from build123d import *

# Parameters (mm, degrees)
SKETCH1_W           = 100
SKETCH1_H           = 100
SKETCH1_R           = 11
BOSS_EXTRUDE1_DEPTH = 12
SKETCH9_W           = 100
SKETCH9_H           = 50
BOSS_EXTRUDE3_DEPTH = 12
CUT_EXTRUDE3_REACH  = 114.446
SKETCH4_R           = 10.5
CUT_EXTRUDE4_REACH  = 114.446
CUT_EXTRUDE5_REACH  = 114.446
SKETCH6_R           = 26
CUT_EXTRUDE6_REACH  = 114.446
CUT_EXTRUDE7_REACH  = 114.446
SKETCH11_R          = 52.045454545
CUT_EXTRUDE8_REACH  = 114.446
SKETCH12_R          = 3


with BuildPart() as part:
    # Sketch1 → Boss-Extrude1 (new body)
    with BuildSketch(Plane(origin=(0, 0, 0), x_dir=(1, 0, 0), z_dir=(0, 1, 0))):
        Rectangle(SKETCH1_W, SKETCH1_H)
        with Locations(Location((0, 0, 0), (0, 0, 270))):
            Circle(SKETCH1_R, mode=Mode.SUBTRACT)
    extrude(amount=BOSS_EXTRUDE1_DEPTH)

    # Sketch9 → Boss-Extrude3 (add)
    with BuildSketch(Plane(origin=(0, 12, 0), x_dir=(1, 0, 0), z_dir=(0, 1, 0))):
        with Locations((0, -75)):
            Rectangle(SKETCH9_W, SKETCH9_H)
    extrude(amount=-BOSS_EXTRUDE3_DEPTH)

    # Sketch4 → Cut-Extrude3 (cut, up to next)
    with BuildSketch(Plane(origin=(0, 12, 0), x_dir=(1, 0, 0), z_dir=(0, 1, 0)), mode=Mode.PRIVATE) as cut_extrude3_sk1:
        with Locations(Location((-36, -20, 0), (0, 0, 270))):
            Circle(SKETCH4_R)
    cut_extrude3_tool1 = extrude(cut_extrude3_sk1.sketch, amount=-CUT_EXTRUDE3_REACH, mode=Mode.PRIVATE) & part.part
    # Sketch4 → Cut-Extrude3 (cut, up to next)
    with BuildSketch(Plane(origin=(0, 12, 0), x_dir=(1, 0, 0), z_dir=(0, 1, 0)), mode=Mode.PRIVATE) as cut_extrude3_sk2:
        with Locations(Location((36, -20, 0), (0, 0, 270))):
            Circle(SKETCH4_R)
    cut_extrude3_tool2 = extrude(cut_extrude3_sk2.sketch, amount=-CUT_EXTRUDE3_REACH, mode=Mode.PRIVATE) & part.part
    add(cut_extrude3_tool1.solids().sort_by_distance((-36, 12, 20))[0], mode=Mode.SUBTRACT)
    add(cut_extrude3_tool2.solids().sort_by_distance((36, 12, 20))[0], mode=Mode.SUBTRACT)

    # Sketch5 → Cut-Extrude4 (cut, up to next)
    with BuildSketch(Plane(origin=(0, 12, 0), x_dir=(1, 0, 0), z_dir=(0, 1, 0)), mode=Mode.PRIVATE) as cut_extrude4_sk1:
        Polygon((-50, 0), (-32, 0), (-32, 18), (32, 18), (32, 0), (50, 0), (50, 50), (-50, 50), align=None)
    cut_extrude4_tool1 = extrude(cut_extrude4_sk1.sketch, amount=-CUT_EXTRUDE4_REACH, mode=Mode.PRIVATE) & part.part
    add(cut_extrude4_tool1.solids().sort_by_distance((0, 12, -29.790021))[0], mode=Mode.SUBTRACT)

    # Sketch6 → Cut-Extrude5 (cut, up to next)
    with BuildSketch(Plane(origin=(0, 12, 0), x_dir=(1, 0, 0), z_dir=(0, 1, 0)), mode=Mode.PRIVATE) as cut_extrude5_sk1:
        with Locations(Location((-0.234960822, -55, 0), (0, 0, 270))):
            Circle(SKETCH6_R)
    cut_extrude5_tool1 = extrude(cut_extrude5_sk1.sketch, amount=-CUT_EXTRUDE5_REACH, mode=Mode.PRIVATE) & part.part
    add(cut_extrude5_tool1.solids().sort_by_distance((-0.234961, 12, 55))[0], mode=Mode.SUBTRACT)

    # Sketch10 → Cut-Extrude6 (cut, up to next)
    with BuildSketch(Plane(origin=(0, 12, 0), x_dir=(1, 0, 0), z_dir=(0, 1, 0)), mode=Mode.PRIVATE) as cut_extrude6_sk1:
        with BuildLine():
            Line((-10.234960822, -88.541019662), (-10.234960822, -100))
            Line((-10.234960822, -100), (-50, -100))
            Line((-50, -100), (-50, -40))
            Line((-50, -40), (-35.234177398, -54.765822602))
            ThreePointArc((-35.234177398, -54.765822602), (-28.367208461, -75.822503278), (-10.234960822, -88.541019662))
        make_face()
    cut_extrude6_tool1 = extrude(cut_extrude6_sk1.sketch, amount=-CUT_EXTRUDE6_REACH, mode=Mode.PRIVATE) & part.part
    # Sketch10 → Cut-Extrude6 (cut, up to next)
    with BuildSketch(Plane(origin=(0, 12, 0), x_dir=(1, 0, 0), z_dir=(0, 1, 0)), mode=Mode.PRIVATE) as cut_extrude6_sk2:
        with BuildLine():
            Line((9.765039178, -88.541019662), (9.765039178, -100))
            Line((9.765039178, -100), (50, -100))
            Line((50, -100), (50, -40))
            Line((50, -40), (34.764245164, -55.235754836))
            ThreePointArc((34.764245164, -55.235754836), (27.756864791, -76.010894766), (9.765039178, -88.541019662))
        make_face()
    cut_extrude6_tool2 = extrude(cut_extrude6_sk2.sketch, amount=-CUT_EXTRUDE6_REACH, mode=Mode.PRIVATE) & part.part
    # Sketch10 → Cut-Extrude6 (cut, up to next)
    with BuildSketch(Plane(origin=(0, 12, 0), x_dir=(1, 0, 0), z_dir=(0, 1, 0)), mode=Mode.PRIVATE) as cut_extrude6_sk3:
        with BuildLine():
            Line((-0.734960822, -80.995191863), (-0.734960822, -100))
            Line((-0.734960822, -100), (0.265039178, -100))
            Line((0.265039178, -100), (0.265039178, -80.995191863))
            ThreePointArc((0.265039178, -80.995191863), (-0.234960822, -81), (-0.734960822, -80.995191863))
        make_face()
    cut_extrude6_tool3 = extrude(cut_extrude6_sk3.sketch, amount=-CUT_EXTRUDE6_REACH, mode=Mode.PRIVATE) & part.part
    add(cut_extrude6_tool1.solids().sort_by_distance((-35.978986, 12, 79.410224))[0], mode=Mode.SUBTRACT)
    add(cut_extrude6_tool2.solids().sort_by_distance((35.780347, 12, 79.379296))[0], mode=Mode.SUBTRACT)
    add(cut_extrude6_tool3.solids().sort_by_distance((-0.234961, 12, 90.499199))[0], mode=Mode.SUBTRACT)

    # Sketch11 → Cut-Extrude7 (cut, up to next)
    with BuildSketch(Plane(origin=(0, 12, 0), x_dir=(1, 0, 0), z_dir=(0, 1, 0)), mode=Mode.PRIVATE) as cut_extrude7_sk1:
        with Locations((0, 41.045454545)):
            Circle(SKETCH11_R)
    cut_extrude7_tool1 = extrude(cut_extrude7_sk1.sketch, amount=-CUT_EXTRUDE7_REACH, mode=Mode.PRIVATE) & part.part
    add(cut_extrude7_tool1.solids().sort_by_distance((0, 12, -41.045455))[0], mode=Mode.SUBTRACT)

    # Sketch12 → Cut-Extrude8 (cut, up to next)
    with BuildSketch(Plane(origin=(0, 12, 0), x_dir=(1, 0, 0), z_dir=(0, 1, 0)), mode=Mode.PRIVATE) as cut_extrude8_sk1:
        with Locations(Location((-15.162534268, -20, 0), (0, 0, 270))):
            Circle(SKETCH12_R)
    cut_extrude8_tool1 = extrude(cut_extrude8_sk1.sketch, amount=-CUT_EXTRUDE8_REACH, mode=Mode.PRIVATE) & part.part
    # Sketch12 → Cut-Extrude8 (cut, up to next)
    with BuildSketch(Plane(origin=(0, 12, 0), x_dir=(1, 0, 0), z_dir=(0, 1, 0)), mode=Mode.PRIVATE) as cut_extrude8_sk2:
        with Locations(Location((14.837465732, -20, 0), (0, 0, 270))):
            Circle(SKETCH12_R)
    cut_extrude8_tool2 = extrude(cut_extrude8_sk2.sketch, amount=-CUT_EXTRUDE8_REACH, mode=Mode.PRIVATE) & part.part
    add(cut_extrude8_tool1.solids().sort_by_distance((-15.162534, 12, 20))[0], mode=Mode.SUBTRACT)
    add(cut_extrude8_tool2.solids().sort_by_distance((14.837466, 12, 20))[0], mode=Mode.SUBTRACT)


solid = part.part
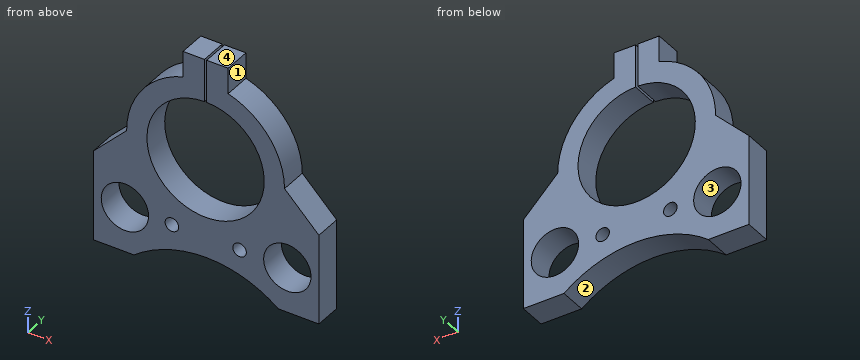
Input: part model. Units: mm. Frame: model coordinates. Face numbers are marked on the shaded views. Round coordinates to 2 decimals unless told otherwise and drop trailing zeros. Order: outer loops, then holes, each group sorted by start corner. A loop starts at its lowest first (then second) coordinate and runs counter-clockwise, first axis right, second up. Notation, with made-up numbers: (10.5, 62.25) - (23.5, 62.25) arc R23 cw to (23.5, 78.25) - close; hole circle Ø1 at (87.5, 23.5). An arc over 180 degrees is marked (long way). Answer as a JSON object with one key per item and string values. Group by question number.
(1) Cut plane A-A (z = 20). Return loops of the section in (x, y).
(2) Cut plane C-C (z = 83). Return loops of the section in (x, y), then the cut area to 3 significant figures.
(3) Draft query along X for the marked faces 1, 2, 3 and 4. Return one class per face: released by +X, released by -X, zero draft, split by the parting line, or undercut.
(4) Cut plane B-B (x = 36). Return loops of the section in (y, z), then the cut area to 3 significant figures.
(5) Material intervals for probe 1 along X at (y, z) = (6.5, 20); probe 2 along Z at (x, y) = (14, 8); probe 3 along X at (y, z) = (0.5, 12.5), sorted ascending. Write a range as from..to.
(6) Cut plane D-D (y = 2.75). Return loops of the section in (x, z), then the cut area to 3 significant figures.
(7) Pin query (flat end, axial travel): P1, Ø4, axis at x = -31.5, y = 10, coming from the +Z side; P2, Ø3, axis at y = 5, z = 53.5, coming from the -X side; P3, Ø5.5, axis at y = 8, z = 92, coming from the -X side. Return the tip coordinate at first contact, or that it passes through.
Here are the results:
{
 "1": {"outline": "(-50, 0) - (-46.5, 0) - (-46.5, 12) - (-50, 12) - close; (-25.5, 0) - (-18.16, 0) - (-18.16, 12) - (-25.5, 12) - close; (-12.16, 0) - (11.84, 0) - (11.84, 12) - (-12.16, 12) - close; (17.84, 0) - (25.5, 0) - (25.5, 12) - (17.84, 12) - close; (46.5, 0) - (50, 0) - (50, 12) - (46.5, 12) - close"},
 "2": {"outline": "(-21.23, 0) - (-0.73, 0) - (-0.73, 12) - (-21.23, 12) - close; (0.27, 0) - (20.77, 0) - (20.77, 12) - (0.27, 12) - close", "area": "492 mm^2"},
 "3": {"face 1": "released by +X", "face 2": "undercut", "face 3": "undercut", "face 4": "zero draft"},
 "4": {"outline": "(0, 0) - (12, 0) - (12, 9.5) - (0, 9.5) - close; (0, 30.5) - (12, 30.5) - (12, 54) - (0, 54) - close", "area": "396 mm^2"},
 "5": {"probe 1": "x = -50..-46.5, -25.5..-18.16, -12.16..11.84, 17.84..25.5, 46.5..50", "probe 2": "z = 9.08..17.12, 22.88..33.24, 76.76..86.97", "probe 3": "x = -50..-43.35, -28.65..28.65, 43.35..50"},
 "6": {"outline": "(-50, 0) - (-32, 0) arc R52.05 cw to (32, 0) - (50, 0) - (50, 40) - (34.76, 55.24) arc R35 ccw to (9.77, 88.54) - (9.77, 100) - (0.27, 100) - (0.27, 81) arc R26 cw (long way) to (-0.73, 81) - (-0.73, 100) - (-10.23, 100) - (-10.23, 88.54) arc R35 ccw to (-35.23, 54.77) - (-50, 40) - close; hole circle Ø21 at (-36, 20); hole circle Ø6 at (-15.16, 20); hole circle Ø6 at (14.84, 20); hole circle Ø21 at (36, 20)", "area": "4,040 mm^2"},
 "7": {"P1": "stops at z = 74.2", "P2": "stops at x = -38", "P3": "stops at x = -10.23"}
}
